Verification items for the finished model (mm, model axes). Face numbers are marked on the shaded views. Round coordinates to 2 decimals unless told otherwise and drop trailing zeros. Loops run counter-clockwise (first coordinate to the right, second up) from the corner with the lowest first, then second, coordinate; pieces in that order, holes last. Notation, with made-up numbers: (84.25, 66.25) - (142.25, 66.25) arc R10 ccw to (142.25, 83.25) - close; hole circle Ø2 at (-23, 39.5). An arc over 180 degrees is marked (long way). Use a Markdown table: item, result. Add a question column.
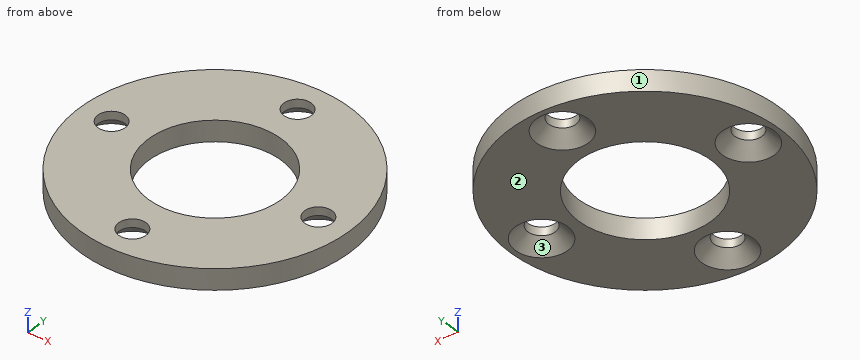
```python
from build123d import *

# Parameters (mm, degrees)
ESQUISSE1_R                  = 32.5
BOSS_EXTRU_1_DEPTH           = 5
R_P_TITION_CIRCULAIRE1_COUNT = 4
ESQUISSE2_R                  = 16
ENL_V_MAT_EXTRU_1_DEPTH      = 6


with BuildPart() as part:
    # Esquisse1 → Boss.-Extru.1 (new body)
    with BuildSketch(Plane.XY):
        Circle(ESQUISSE1_R)
    extrude(amount=BOSS_EXTRU_1_DEPTH)

    # Esquisse5 → Fraisage pour vis à tête fraisée M61 (revolve, cut)
    with BuildSketch(Plane(origin=(0, -25, 0), x_dir=(0, 1, 0), z_dir=(1, 0, 0))):
        Polygon((0, 0), (0, 5), (3.3, 5), (3.3, 3), (6.3, 0), align=None)
    fraisage_pour_vis_t_te_frais_e_m61 = revolve(axis=Axis((0, -25, -6.35), (0, 0, 1)), mode=Mode.SUBTRACT)

    # Répétition circulaire1: Fraisage pour vis à tête fraisée M61 ×4 about axis
    r_p_tition_circulaire1_axis = Axis((0, 0, 0), (0, 0, 1))
    for i in range(1, R_P_TITION_CIRCULAIRE1_COUNT):
        add(fraisage_pour_vis_t_te_frais_e_m61.rotate(r_p_tition_circulaire1_axis, i * 360 / R_P_TITION_CIRCULAIRE1_COUNT), mode=Mode.SUBTRACT)

    # Esquisse2 → Enlèv. mat.-Extru.1 (cut, through all)
    with BuildSketch(Plane.XY.offset(5)):
        Circle(ESQUISSE2_R)
    extrude(amount=-ENL_V_MAT_EXTRU_1_DEPTH, mode=Mode.SUBTRACT)


solid = part.part
```
Q1. Section check B-B on y = 25. Record the cut outline in (x, z), plus the area to 3 significant figures.
Q2. Release check for a two-part mould opening along Y. For the marked faces 1, 2 and 3 record: +Y half, -Y half, draft (parallel to the pull), parting line (faces both ways), or undercut.
Q3. Section check A-A on x = 0. Record the cut outline in (y, z).
Q4. Thickness scan on line 1 along X through (y, z) = (-4.5, 0.25); line 2 along Y through (x, z) = (-1, 3.2); line 3 along X through (y, z) = (-9, 1.6). Record the ranges inside material, lowest first.
Q5. Section check C-C on x = 10.5. Record the cut outline in (y, z), plus the area to 3 significant figures.
Q6. Go/stop test with flat-tipped pins: pin 1 Ø3 at (x, z) = (12, 1) entering from -Y; pin 2 Ø5.5 at (x, y) = (0, 25) entering from -Z; pin 3 Ø10 at (x, y) = (-17.5, -22.5) entering from -Z; pin 4 Ø2 at (y, z) = (-14, 2) entering from -X. Record where each tip stops, or that it passes through.
Q7. Section check D-D on y = -11.5. Record the cut outline in (x, z), plus the area to 3 significant figures.
Determined:
| question | item | result |
|---|---|---|
| 1 | outline | (-20.77, 0) - (-6.3, 0) - (-3.3, 3) - (-3.3, 5) - (-20.77, 5) - close; (3.3, 3) - (6.3, 0) - (20.77, 0) - (20.77, 5) - (3.3, 5) - close |
| 1 | area | 166 mm² |
| 2 | face 1 | parting line |
| 2 | face 2 | draft |
| 2 | face 3 | undercut |
| 3 | outline | (-32.5, 0) - (-31.3, 0) - (-28.3, 3) - (-28.3, 5) - (-32.5, 5) - close; (-21.7, 3) - (-18.7, 0) - (-16, 0) - (-16, 5) - (-21.7, 5) - close; (16, 0) - (18.7, 0) - (21.7, 3) - (21.7, 5) - (16, 5) - close; (28.3, 3) - (31.3, 0) - (32.5, 0) - (32.5, 5) - (28.3, 5) - close |
| 4 | line 1 | x = -32.19 to -29.04, -20.96 to -15.35, 15.35 to 20.96, 29.04 to 32.19 |
| 4 | line 2 | y = -32.48 to -28.14, -21.86 to -15.97, 15.97 to 21.86, 28.14 to 32.48 |
| 4 | line 3 | x = -31.23 to -13.23, 13.23 to 31.23 |
| 5 | outline | (-30.76, 0) - (-12.07, 0) - (-12.07, 5) - (-30.76, 5) - close; (12.07, 0) - (30.76, 0) - (30.76, 5) - (12.07, 5) - close |
| 5 | area | 187 mm² |
| 6 | pin 1 | stops at y = -30.76 |
| 6 | pin 2 | passes through |
| 6 | pin 3 | stops at z = 0 |
| 6 | pin 4 | stops at x = -29.79 |
| 7 | outline | (-30.4, 0) - (-11.12, 0) - (-11.12, 5) - (-30.4, 5) - close; (11.12, 0) - (30.4, 0) - (30.4, 5) - (11.12, 5) - close |
| 7 | area | 193 mm² |
